```python
from build123d import *

# Parameters (mm, degrees)
F0_R     = 6.35
F1_DEPTH = 25.4
F2_W     = 70.0848072124
F2_H     = 25.4
F3_DEPTH = 50.8
F5_DEPTH = 25.4
F6_R     = 4.445
F7_DEPTH = 127
F8_R     = 12.69999


# Not quite as in the source:
# - a fillet or chamfer is up to 0.001 mm smaller than in the source, because OpenCascade refuses the exact size


with BuildPart() as f1:
    # F0 (on Front) → F1 (new body)
    with BuildSketch(Plane.XZ):
        with BuildLine():
            Line((-54.7069231111, -19.05), (50.7348023818, -19.05))
            ThreePointArc((50.7348023818, -19.05), (69.7848023818, 0), (50.7348023818, 19.05))
            Line((50.7348023818, 19.05), (-54.7069231111, 19.05))
            ThreePointArc((-54.7069231111, 19.05), (-73.7569231111, 0), (-54.7069231111, -19.05))
        make_face()
        with Locations((-54.7069231111, 0)):
            Circle(F0_R, mode=Mode.SUBTRACT)
        with Locations((50.7348023818, 0)):
            Circle(F0_R, mode=Mode.SUBTRACT)
    extrude(amount=F1_DEPTH)

    # F2 (on face) → F3 (join)
    with BuildSketch(Plane.XZ.offset(25.4)):
        Rectangle(F2_W, F2_H)
    extrude(amount=F3_DEPTH)

    # F4 (on face) → F5 (cut)
    with BuildSketch(Plane(origin=(0, 0, -12.7), x_dir=(1, 0, 0), z_dir=(0, 0, -1))):
        with BuildLine():
            Line((22.1503823996, 76.2), (-22.2996176004, 76.2))
            Line((-22.2996176004, 76.2), (-22.2996176004, 48.7618595362))
            ThreePointArc((-22.2996176004, 48.7618595362), (1.2899395164, 26.4995819984), (22.1503823996, 51.3374186365))
            Line((22.1503823996, 51.3374186365), (22.1503823996, 76.2))
        make_face()
    extrude(amount=-F5_DEPTH, mode=Mode.SUBTRACT)

    # F6 (on face) → F7 (cut)
    with BuildSketch(Plane(origin=(-35.0424036062, 0, 0), x_dir=(0, -1, 0), z_dir=(-1, 0, 0))):
        with Locations((63.5453920611, 0)):
            Circle(F6_R)
    extrude(amount=-F7_DEPTH, mode=Mode.SUBTRACT)

    # F8 (radius 12.7 in the source; OpenCascade refuses exactly that, so slightly less here)
    f8_edges = [f1.edges().sort_by_distance(p)[0] for p in [
        (-28.671011, -76.2, 12.7),
        (-28.671011, -76.2, -12.7),
        (28.596393, -76.2, 12.7),
        (28.596393, -76.2, -12.7),
    ]]
    fillet(f8_edges, radius=F8_R)


solid = f1.part
```
Part model, mm, in its own coordinate system. A direction names the side the tool comes from. Round coordinates to 2 decimals unless told otherwise and drop trailing zeros. Loops run counter-clockwise (first coordinate to the right, second up) from the corner with the lowest first, then second, coordinate; pieces in that order, holes last.
1. Two-plate mould, pull along Y, no slides. Class faces 1 (the face through (28.506, -67.651, -1.702)), 2 (the face through (-8, -27, 12.7)), 3 (the face through (-3, 0, 0)), 4 (the face through (28.69, -72.38, 9.08)): pulls with the +Y half, pulls with the -Y half, needs draft (parallel to the pull), parting line crosses it, or undercut.
Solutions:
face 1: undercut
face 2: needs draft
face 3: pulls with the +Y half
face 4: pulls with the -Y half
2. Slice it at C-C (x = 0). Give the cut face in (y, z).
Solutions:
outline: (-26.46, -12.7) - (-25.4, -12.7) - (-25.4, -19.05) - (0, -19.05) - (0, 19.05) - (-25.4, 19.05) - (-25.4, 12.7) - (-26.46, 12.7) - close
3. Slice it at D-D (z = 10). Give the cut face in (x, y).
Solutions:
outline: (-70.92, -25.4) - (-35.04, -25.4) - (-35.04, -71.33) - (-22.3, -71.33) - (-22.3, -48.76) arc R22.3 cw (long way) to (22.15, -51.34) - (22.15, -71.33) - (35.04, -71.33) - (35.04, -25.4) - (66.95, -25.4) - (66.95, 0) - (-70.92, 0) - close
4. Flat gauge pins, fed straight in: pin 1 (1.5 mm diameter, centred on x = 47, z = 11.5, fed in from -Y); pin 2 (5 mm diameter, centred on x = 20.5, y = -52.5, fed in from -Z); pin 3 (12.5 mm diameter, centred on y = -59, z = 3.5, fed in from -X). Where does each tip first touch, or does it go through?
Solutions:
pin 1: stops at y = -25.4
pin 2: stops at z = -12.7
pin 3: stops at x = -35.04
5. Drill centre lines: line 1 along X through (y, z) = (-9, -0.5); line 2 along X through (y, z) = (-51.5, -8); line 3 along X through (y, z) = (-48.5, -11). Where is each one in solid material? Low to high.
Solutions:
line 1: x = -73.75 to -61.04, -48.38 to 44.4, 57.07 to 69.78
line 2: x = -35.04 to -22.3, 22.15 to 35.04
line 3: x = -35.04 to -22.3, 22.3 to 35.04
6. 3-axis set-ups, long thin cutter, end or side, ignore diameter. For faces 5 (the face through (-8, -27, -12.7)), 6 (the face through (22.15, -58, 0)), 7 (the face through (-35.042, -50, 0)), 8 (the face through (-28.76, -67.651, -1.702)): which of +Z, -Z, +X, -X, +Y, -Y reach the whole face in a straight line?
Solutions:
face 5: -Z, +X, -X, -Y
face 6: +Z, -Z, -Y
face 7: +Z, -Z, -X, -Y
face 8: +X, -X
7. Slice it at A-A (y = -55). Give the cut face in (x, z), and give its area (3 significant figures).
Solutions:
outline: (-35.04, -12.7) - (-22.3, -12.7) - (-22.3, 12.7) - (-35.04, 12.7) - close; (22.15, -12.7) - (35.04, -12.7) - (35.04, 12.7) - (22.15, 12.7) - close
area: 651 mm2
